from build123d import *

# Parameters (mm, degrees)
F0_W     = 25
F0_H     = 25
F0_W_2   = 21
F0_H_2   = 21
F1_DEPTH = 270
F2_W     = 25
F2_H     = 12.5
F3_DEPTH = 25.001


with BuildPart() as f1:
    # F0 (on Right) → F1 (new body)
    with BuildSketch(Plane.YZ):
        with Locations((12.5, 12.5)):
            Rectangle(F0_W, F0_H)
        with Locations((12.5, 12.5)):
            Rectangle(F0_W_2, F0_H_2, mode=Mode.SUBTRACT)
    extrude(amount=F1_DEPTH)

    # F2 (on face) → F3 (cut, through all)
    with BuildSketch(Plane.XY.offset(25)):
        with Locations((135, 18.75)):
            Rectangle(F2_W, F2_H)
    extrude(amount=-F3_DEPTH, mode=Mode.SUBTRACT)


solid = f1.part
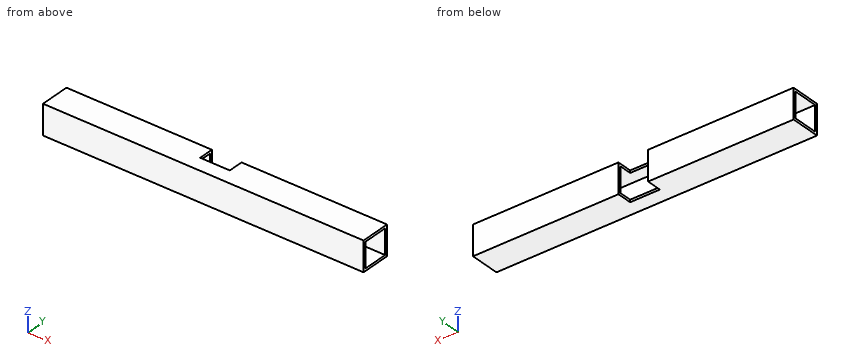
For this review, take the finished solid that the model builds, in its own axes (mm). Round coordinates to 2 decimals unless told otherwise and drop trailing zeros. Write each loop counter-clockwise with the first axis right and the second up, starting at its lowest first coordinate (ties: lowest second). Pieces come first, ordered by that corner, then holes. Notation, with made-up numbers: (9.5, 38.25) - (17.5, 38.25) arc R25 cw to (17.5, 54.25) - close; hole circle Ø1 at (69.25, -26). An arc over 180 degrees is marked (long way). Use a Markdown table: item, result.
Q1. We need section A-A (z = 19). Give the boundary of the cut face in (x, y), plus the area to 3 significant figures.
Derived:
| item | result |
|---|---|
| outline | (0, 0) - (270, 0) - (270, 2) - (0, 2) - close; (0, 23) - (122.5, 23) - (122.5, 25) - (0, 25) - close; (147.5, 23) - (270, 23) - (270, 25) - (147.5, 25) - close |
| area | 1,030 mm2 |
Q2. We need section B-B (y = 19.5). Give the boundary of the cut face in (x, z).
Derived:
| item | result |
|---|---|
| outline | (0, 0) - (122.5, 0) - (122.5, 2) - (0, 2) - close; (0, 23) - (122.5, 23) - (122.5, 25) - (0, 25) - close; (147.5, 0) - (270, 0) - (270, 2) - (147.5, 2) - close; (147.5, 23) - (270, 23) - (270, 25) - (147.5, 25) - close |
Q3. We need section C-C (x = 46.5). Give the boundary of the cut face in (y, z).
Derived:
| item | result |
|---|---|
| outline | (0, 0) - (25, 0) - (25, 25) - (0, 25) - close; hole (2, 2) - (23, 2) - (23, 23) - (2, 23) - close |
Q4. Wall thickness on line 1 along Y through (x, z) = (209, 6); line 2 along Y through (x, z) = (144, 10): over which ranges is each line inside the solid? List them lowest first.
Derived:
| item | result |
|---|---|
| line 1 | y = 0 to 2, 23 to 25 |
| line 2 | y = 0 to 2 |
Q5. Clearance check with flat-ended pins moving along their axes: pin 1 (10 mm diameter, centred on x = 200, y = 19.5, fed in from -Z); pin 2 (1.5 mm diameter, centred on x = 134, z = 18.5, fed in from +Y); pin 3 (2 mm diameter, centred on x = 133.5, z = 1.5, fed in from +Y); pin 4 (10 mm diameter, centred on y = 16.5, z = 12, fed in from -X). State where each tip first meets the part, or that it passes through.
Derived:
| item | result |
|---|---|
| pin 1 | stops at z = 0 |
| pin 2 | stops at y = 2 |
| pin 3 | stops at y = 12.5 |
| pin 4 | passes through |
Q6. We need section D-D (x = 134.5). Give the boundary of the cut face in (y, z), plus the area to 3 significant figures.
Derived:
| item | result |
|---|---|
| outline | (0, 0) - (12.5, 0) - (12.5, 2) - (2, 2) - (2, 23) - (12.5, 23) - (12.5, 25) - (0, 25) - close |
| area | 92.0 mm2 |
